```python
from build123d import *

# Parameters (mm, degrees)
F0_W     = 515
F0_H     = 68
F1_DEPTH = 10
F2_R     = 3.5
F2_R_2   = 6.25
F3_DEPTH = 10.001
F4_W     = 17.5
F4_H     = 49
F4_W_2   = 17
F5_DEPTH = 10.001
F4_W_3   = 29
F4_H_2   = 47.3
F6_DEPTH = 10.001
F7_R     = 4
F8_R     = 6


with BuildPart() as f1:
    # F0 (on Front) → F1 (new body)
    with BuildSketch(Plane.XZ):
        with Locations((257.5, -34)):
            Rectangle(F0_W, F0_H)
    extrude(amount=F1_DEPTH)

    # F2 (on face) → F3 (cut, through all)
    with BuildSketch(Plane.XZ.offset(10)):
        with Locations((7.5, -8.5)):
            Circle(F2_R)
        with Locations((507.5, -8.5)):
            Circle(F2_R)
        with Locations((10.5, -30.75)):
            Circle(F2_R_2)
        with Locations((51, -30.75)):
            Circle(F2_R_2)
        with Locations((128, -30.75)):
            Circle(F2_R_2)
        with Locations((258, -30.75)):
            Circle(F2_R_2)
        with Locations((388, -30.75)):
            Circle(F2_R_2)
        with Locations((463.5, -30.75)):
            Circle(F2_R_2)
        with Locations((504, -30.75)):
            Circle(F2_R_2)
    extrude(amount=-F3_DEPTH, mode=Mode.SUBTRACT)

    # F4 (on face) → F5 (cut, through all)
    with BuildSketch(Plane.XZ.offset(10)):
        with Locations((30.25, -37.5)):
            Rectangle(F4_W, F4_H)
        with Locations((482.5, -37.5)):
            Rectangle(F4_W_2, F4_H)
    extrude(amount=-F5_DEPTH, mode=Mode.SUBTRACT)

    # F4 (on face) → F6 (cut, through all)
    with BuildSketch(Plane.XZ.offset(10)):
        with Locations((90, -31.65)):
            Rectangle(F4_W_3, F4_H_2)
        with Locations((156.5, -31.65)):
            Rectangle(F4_W_3, F4_H_2)
        with Locations((359, -31.65)):
            Rectangle(F4_W_3, F4_H_2)
        with Locations((425, -31.65)):
            Rectangle(F4_W_3, F4_H_2)
    extrude(amount=-F6_DEPTH, mode=Mode.SUBTRACT)

    # F7
    f7_edges = [f1.edges().sort_by_distance(p)[0] for p in [
        (21.5, -5, -13),
        (21.5, -5, -62),
        (39, -5, -62),
        (39, -5, -13),
        (491, -5, -13),
        (474, -5, -13),
        (474, -5, -62),
        (491, -5, -62),
    ]]
    fillet(f7_edges, radius=F7_R)

    # F8
    f8_edges = [f1.edges().sort_by_distance(p)[0] for p in [
        (410.5, -5, -8),
        (439.5, -5, -8),
        (75.5, -5, -8),
        (104.5, -5, -8),
        (171, -5, -8),
        (75.5, -5, -55.3),
        (142, -5, -55.3),
        (142, -5, -8),
        (171, -5, -55.3),
        (104.5, -5, -55.3),
        (439.5, -5, -55.3),
        (373.5, -5, -55.3),
        (410.5, -5, -55.3),
        (344.5, -5, -55.3),
        (373.5, -5, -8),
        (344.5, -5, -8),
    ]]
    fillet(f8_edges, radius=F8_R)


solid = f1.part
```
Model file for the job. Use its own axes, mm. Give positions to 0.01 mm unless a question says otherwise; leave off trailing zeros. Loops run counter-clockwise (first coordinate to the right, second up) from the corner with the lowest first, then second, coordinate; pieces in that order, holes last. Notation, with made-up numbers: (1.5, -24) -> (31.5, -24) arc R18 ccw to (31.5, -20) -> close; hole circle Ø3 at (56.25, -20). An arc over 180 degrees is marked (long way). Use CSV: the item, a comma, the result in double quotes. Start each with the question number.
1) Slice it at C-C on y = -4.25. Give the number of separate pieces and of enclosed holes in the cut face, plus the area to 3 significant figures.
2) Slice it at B-B on x = 388. Give the cut face in (y, z).
3) Slice it at A-A on z = -41.5. Give the cut face in (x, y), plus the area to 4 significant figures.
4) Wall check: line 1 (X direction, y = -8.5, z = -58); line 2 (Z direction, x = 507.5, y = -5.5); line 3 (Z direction, x = 31, y = -4.25). Give the ranges that are in metal, low to high.
5) Mould opens along X. For faces 1 (the cylindrical face through (134, -5, -29)), 2 (the flat face through (373.5, -5, -32)), 3 (the flat face through (254, -5, 0)) say: released by +X, released by -X, zero draft, split by the parting line, or undercut.
Computed values:
1,separate pieces,"1"
1,enclosed holes,"15"
1,area,"27,100 mm^2"
2,outline,"(-10, -68) -> (0, -68) -> (0, -37) -> (-10, -37) -> close; (-10, -24.5) -> (0, -24.5) -> (0, 0) -> (-10, 0) -> close"
3,outline,"(0, -10) -> (21.5, -10) -> (21.5, 0) -> (0, 0) -> close; (39, -10) -> (75.5, -10) -> (75.5, 0) -> (39, 0) -> close; (104.5, -10) -> (142, -10) -> (142, 0) -> (104.5, 0) -> close; (171, -10) -> (344.5, -10) -> (344.5, 0) -> (171, 0) -> close; (373.5, -10) -> (410.5, -10) -> (410.5, 0) -> (373.5, 0) -> close; (439.5, -10) -> (474, -10) -> (474, 0) -> (439.5, 0) -> close; (491, -10) -> (515, -10) -> (515, 0) -> (491, 0) -> close"
3,area,"3,645 mm^2"
4,line 1,"x = 0 to 21.5, 39 to 474, 491 to 515"
4,line 2,"z = -68 to -35.93, -25.57 to -12, -5 to 0"
4,line 3,"z = -68 to -62, -13 to 0"
5,face 1,"undercut"
5,face 2,"undercut"
5,face 3,"zero draft"
